from build123d import *

# Parameters (mm, degrees)
F1_DEPTH = 75
F2_R     = 13.5
F3_DEPTH = 20
F5_DEPTH = 55.001
F7_DEPTH = 55.001


with BuildPart() as f1:
    # F0 (on Top) → F1 (new body)
    with BuildSketch(Plane.XY):
        with BuildLine():
            Line((0, 40), (0, 0))
            Line((0, 0), (15, 0))
            Line((15, 0), (15, 14.675536))
            ThreePointArc((15, 14.675536), (22.822899, 21.507602), (30, 14))
            Line((30, 14), (30, 0))
            Line((30, 0), (55, 0))
            Line((55, 0), (55, 25))
            Line((55, 25), (75, 25))
            Line((75, 25), (75, 34.041284))
            ThreePointArc((75, 34.041284), (67.415432, 49.721114), (50.414294, 53.508469))
            Line((50.414294, 53.508469), (0, 40))
        make_face()
    extrude(amount=F1_DEPTH)

    # F2 (on face) → F3 (join)
    with BuildSketch(Plane.XY.offset(75)):
        with Locations((59.202516, 39)):
            Circle(F2_R)
    extrude(amount=F3_DEPTH)

    # F4 (on face) → F5 (cut, through all)
    with BuildSketch(Plane.YZ.offset(55)):
        Polygon((20, 45), (0, 55), (0, 42.03419), align=None)
    extrude(amount=-F5_DEPTH, mode=Mode.SUBTRACT)

    # F6 (on face) → F7 (cut, through all)
    with BuildSketch(Plane.YZ.offset(55)):
        Polygon((20, 0), (0, 20), (0, 0), align=None)
    extrude(amount=-F7_DEPTH, mode=Mode.SUBTRACT)


solid = f1.part
Geometry check sheet. Reference: the model listing, model coordinates, mm. A direction names the side the tool comes from. Round coordinates to 2 decimals unless told otherwise and drop trailing zeros. Order: outer loops, then holes, each group sorted by start corner. A loop starts at its lowest first (then second) coordinate and runs counter-clockwise, first axis right, second up. Notation, with made-up numbers: M 17.5,83.5 L 41.5,83.5 A24 ccw 41.5,114.5 Z; hole C 30,40 d2. An arc over 180 degrees is marked long. Answer in a Markdown table with one row per item. Add a question column.
Item 1: Sectioned sample at D-D, the plane z = 51.5. Enter the section's corners in (x, y), plus the area to 3 significant figures.
Item 2: Sectioned sample at A-A, the plane z = 14.5. Enter the section's corners in (x, y), plus the area to 3 significant figures.
Item 3: Draft check along Z on faces 1 (the face through (29, 27, 75)), 2 (the face through (41, 10, 50)), 3 (the face through (30, 7, 64)). Enter one of: released by +Z, released by -Z, zero draft, split by the parting line, or undercut.
Item 4: Depth check by flat-ended pin: pin 1 Ø2 at (x, y) = (51, 24) entering from +Z; pin 2 Ø4.5 at (y, z) = (5.5, 23.5) entering from +X. Enter the tip coordinate at first touch or a pass-through.
Item 5: Sectioned sample at C-C, the plane x = 60. Enter the section's corners in (y, z), plus the area to 3 significant figures.
Item 6: Sectioned sample at B-B, the plane y = 7. Enter the section's corners in (x, z).
Item 7: Set-up check for faces 4 (the face through (65, 25, 37)), 5 (the face through (15, 7, 64)), 6 (the face through (0, 20, 37)): record each of +Z, -Z, +X, -X, +Y, -Y from which the full face is reachable in a straight line by a thin tool's end or side.
Item 8: Material ranges on L1, parallel to Y at x = 54, z = 57; L2, parallel to Z at x = 12, y = 43; L3, parallel to X at y = 23.5, z = 36.5, recorded low to high. Write a range as [from, to].
Filled in:
| question | item | result |
|---|---|---|
| 1 | outline | M 0,7 L 15,7 L 15,14.68 A7.52 cw 30,14 L 30,7 L 55,7 L 55,25 L 75,25 L 75,34.04 A20 ccw 50.41,53.51 L 0,40 Z |
| 1 | area | 2,520 mm² |
| 2 | outline | M 0,5.5 L 15,5.5 L 15,14.68 A7.52 cw 30,14 L 30,5.5 L 55,5.5 L 55,25 L 75,25 L 75,34.04 A20 ccw 50.41,53.51 L 0,40 Z |
| 2 | area | 2,580 mm² |
| 3 | face 1 | released by +Z |
| 3 | face 2 | undercut |
| 3 | face 3 | zero draft |
| 4 | pin 1 | stops at z = 75 |
| 4 | pin 2 | stops at x = 55 |
| 5 | outline | M 25,0 L 53.41,0 L 53.41,75 L 52.48,75 L 52.48,95 L 25.52,95 L 25.52,75 L 25,75 Z |
| 5 | area | 2,670 mm² |
| 6 | outline | M 0,13 L 15,13 L 15,43.07 L 0,43.07 Z; M 0,51.5 L 15,51.5 L 15,75 L 0,75 Z; M 30,13 L 55,13 L 55,43.07 L 30,43.07 Z; M 30,51.5 L 55,51.5 L 55,75 L 30,75 Z |
| 7 | face 4 | +Z, -Z, +X, -Y |
| 7 | face 5 | +Z, -Z, -Y |
| 7 | face 6 | +Z, -Z, -X, +Y, -Y |
| 8 | L1 | y = [0, 54.02] |
| 8 | L2 | z = [0, 75] |
| 8 | L3 | x = [0, 55] |
